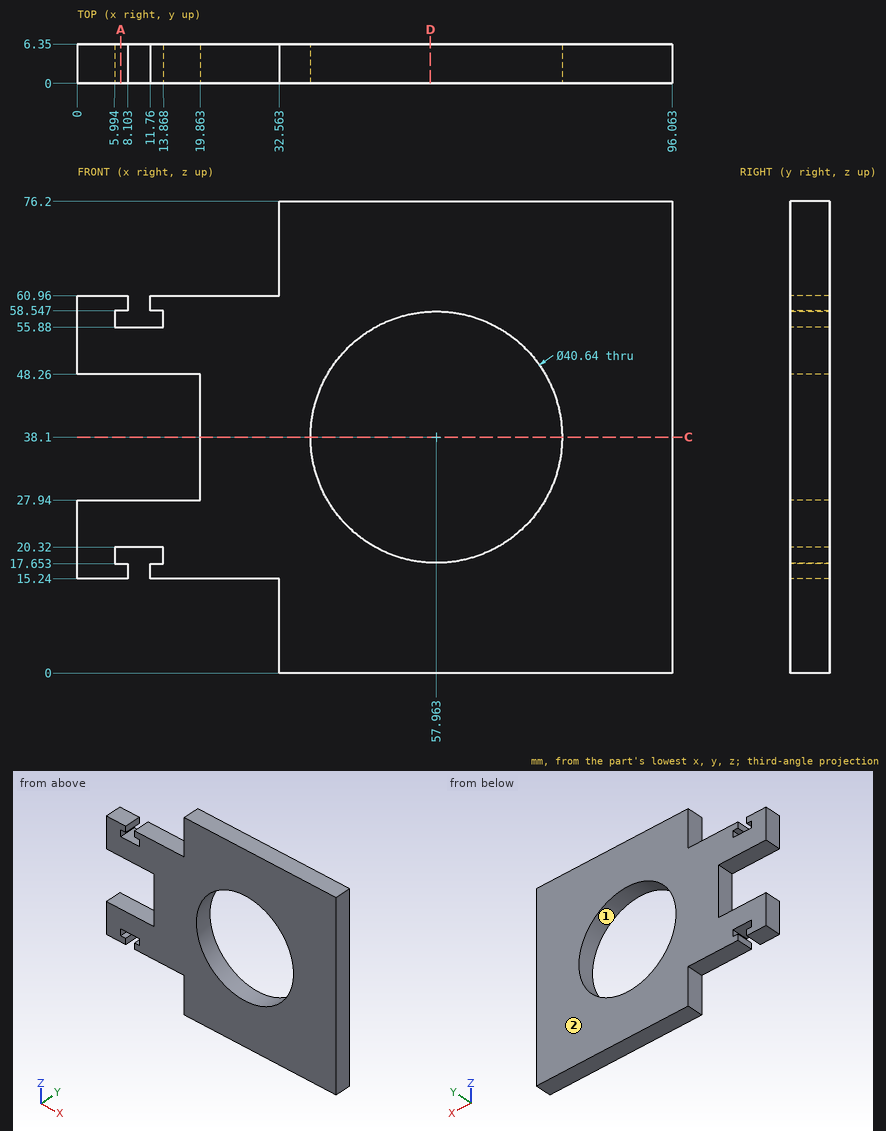
Answer from the drawing. Dimensions are ordinates in mm from the lowest x, y and z of the part. Coordinates: 2 decimals unless noted, no trailing zeros. Loops run counter-clockwise (first coordinate to the right, second up) from the corner with the lowest first, then second, coordinate; pieces in that order, holes last. Notation, with made-up numbers: (19.5, -15.5) -> (53.5, -15.5) arc R11 ccw to (53.5, -4.5) -> close; hole circle Ø6 at (-16, 58). An arc over 180 degrees is marked (long way). Return JSON: item names as keys, results as strings.
Item 1: Find the intervals of material crossed by probe 1 along Z at (x, y) = (7.5, 3); probe 2 along X at (y, z) = (4, 38.1); probe 3 along X at (y, z) = (4.5, 66.5), in increasing order.
Answers:
{"probe 1": "z = 15.24 to 17.65, 20.32 to 27.94, 48.26 to 55.88, 58.55 to 60.96", "probe 2": "x = 19.86 to 37.64, 78.28 to 96.06", "probe 3": "x = 32.56 to 96.06"}
Item 2: Find section D-D (x = 57). Determine the outline of the cut face in (y, z).
Answers:
{"outline": "(0, 0) -> (6.35, 0) -> (6.35, 17.8) -> (0, 17.8) -> close; (0, 58.4) -> (6.35, 58.4) -> (6.35, 76.2) -> (0, 76.2) -> close"}
Item 3: Find section A-A (x = 7). Determine the outline of the cut face in (y, z).
Answers:
{"outline": "(0, 15.24) -> (6.35, 15.24) -> (6.35, 17.65) -> (0, 17.65) -> close; (0, 20.32) -> (6.35, 20.32) -> (6.35, 27.94) -> (0, 27.94) -> close; (0, 48.26) -> (6.35, 48.26) -> (6.35, 55.88) -> (0, 55.88) -> close; (0, 58.55) -> (6.35, 58.55) -> (6.35, 60.96) -> (0, 60.96) -> close"}
Item 4: Flat-ended cylindrical pins translate along their axes: P1, Ø2, axis at x = 18.5, y = 3.5, coming from the -Z side; P2, Ø1.7, axis at x = 13, y = 2, coming from the +Z side. Find the tip coordinate at first contact, or state that the pin passes through.
Answers:
{"P1": "stops at z = 15.24", "P2": "stops at z = 60.96"}
Item 5: Find section C-C (z = 38.1). Determine the outline of the cut face in (x, y).
Answers:
{"outline": "(19.86, 0) -> (37.64, 0) -> (37.64, 6.35) -> (19.86, 6.35) -> close; (78.28, 0) -> (96.06, 0) -> (96.06, 6.35) -> (78.28, 6.35) -> close"}
Item 6: For a pull along Z with two mould halves and no side action, classify the marked faces 1 and 2 as +Z half, -Z half, draft (parallel to the pull), parting line (faces both ways), or undercut.
Answers:
{"face 1": "undercut", "face 2": "draft"}
